Input: dimensioned drawing with shaded views. Units: mm. Origin: part minimum x, y, z. A direction names the side the tool comes from. Coordinates: 2 decimals unless noted, no trailing zeros. Loops run counter-clockwise (first coordinate to the right, second up) from the corner with the lowest first, then second, coordinate; pieces in that order, holes last.
Item 1: Reachability of the marked faces 1 and 2 from +Z, -Z, +X, -X, +Y, -Y: full face, straight path, thin tool, end or side. Return the list, or none.
Item 2: Section A-A on y = 50. Return loops of the section in (x, z), and give its area (3 significant figures).
Item 3: Section D-D on z = 78.5. Return loops of the section in (x, y), and give its area (3 significant figures).
Item 4: Contact query for flat-ended pins moving along their axis: P1, Ø1.5, axis at x = 23, y = 39, coming from the +Z side; P2, Ø2.5, axis at y = 50, z = 47.221, coming from the +X side. Output: stop coordinate, or through.
Item 5: Ray query, line 1 along Z through (x, y) = (1.05, 50); line 2 along Y through (x, z) = (60, 86). Return the intervals inside material, ascending.
Item 6: Section C-C on x = 56.5. Return loops of the section in (y, z), and give its area (3 significant figures).
Item 7: Section B-B on z = 57. Return loops of the section in (x, y), and give its area (3 significant figures).
Item 8: Pull-direction query (Y, two-part tool) for the marked faces 3, 4, 5 and 6; classes: released by +Y, released by -Y, zero draft, split by the parting line, or undercut.
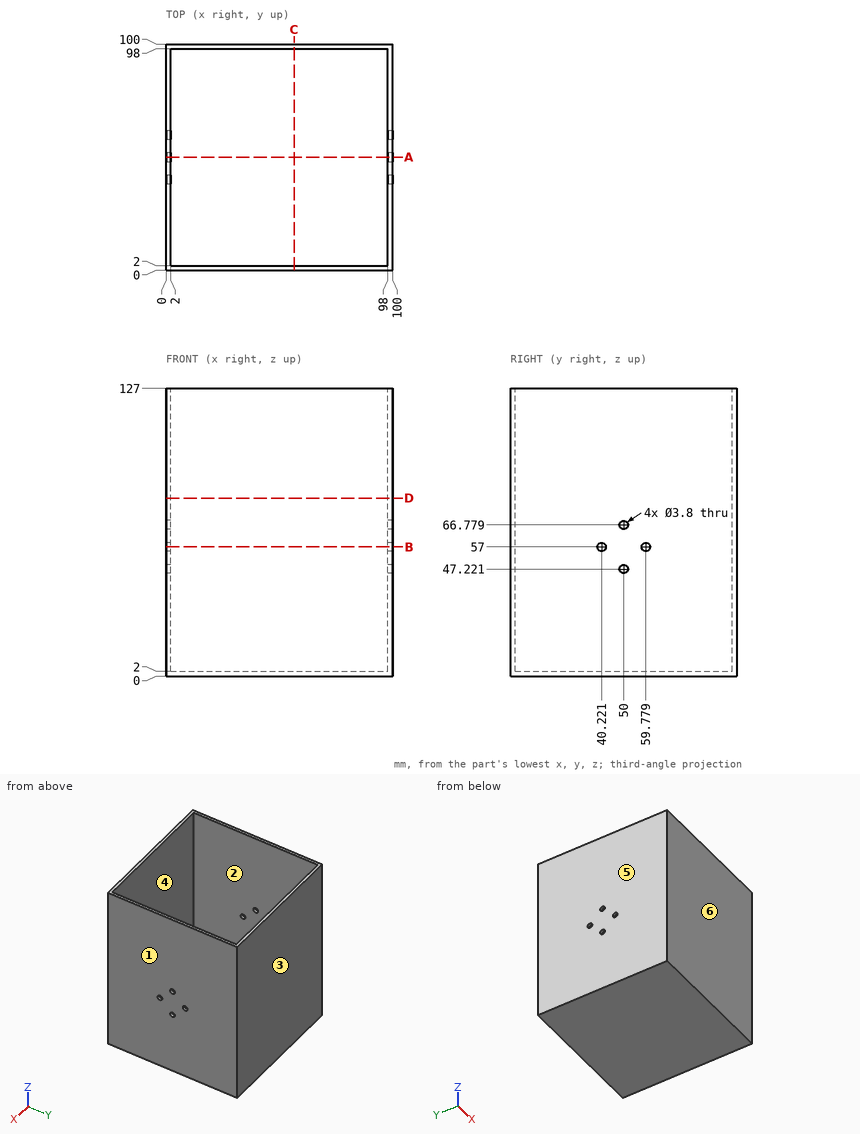
Results found:
1. face 1: +Z, -Z, +X, +Y, -Y
1. face 2: +Z
2. outline: (0, 0) - (100, 0) - (100, 45.32) - (98, 45.32) - (98, 2) - (2, 2) - (2, 45.32) - (0, 45.32) - close; (0, 49.12) - (2, 49.12) - (2, 64.88) - (0, 64.88) - close; (0, 68.68) - (2, 68.68) - (2, 127) - (0, 127) - close; (98, 49.12) - (100, 49.12) - (100, 64.88) - (98, 64.88) - close; (98, 68.68) - (100, 68.68) - (100, 127) - (98, 127) - close
2. area: 670 mm2
3. outline: (0, 0) - (100, 0) - (100, 100) - (0, 100) - close; hole (2, 2) - (98, 2) - (98, 98) - (2, 98) - close
3. area: 784 mm2
4. P1: stops at z = 2
4. P2: passes through
5. line 1: z = 0 to 45.32, 49.12 to 64.88, 68.68 to 127
5. line 2: y = 0 to 2, 98 to 100
6. outline: (0, 0) - (100, 0) - (100, 127) - (98, 127) - (98, 2) - (2, 2) - (2, 127) - (0, 127) - close
6. area: 700 mm2
7. outline: (0, 0) - (100, 0) - (100, 38.32) - (98, 38.32) - (98, 2) - (2, 2) - (2, 38.32) - (0, 38.32) - close; (0, 42.12) - (2, 42.12) - (2, 57.88) - (0, 57.88) - close; (0, 61.68) - (2, 61.68) - (2, 98) - (98, 98) - (98, 61.68) - (100, 61.68) - (100, 100) - (0, 100) - close; (98, 42.12) - (100, 42.12) - (100, 57.88) - (98, 57.88) - close
7. area: 754 mm2
8. face 3: released by +Y
8. face 4: undercut
8. face 5: zero draft
8. face 6: released by -Y
